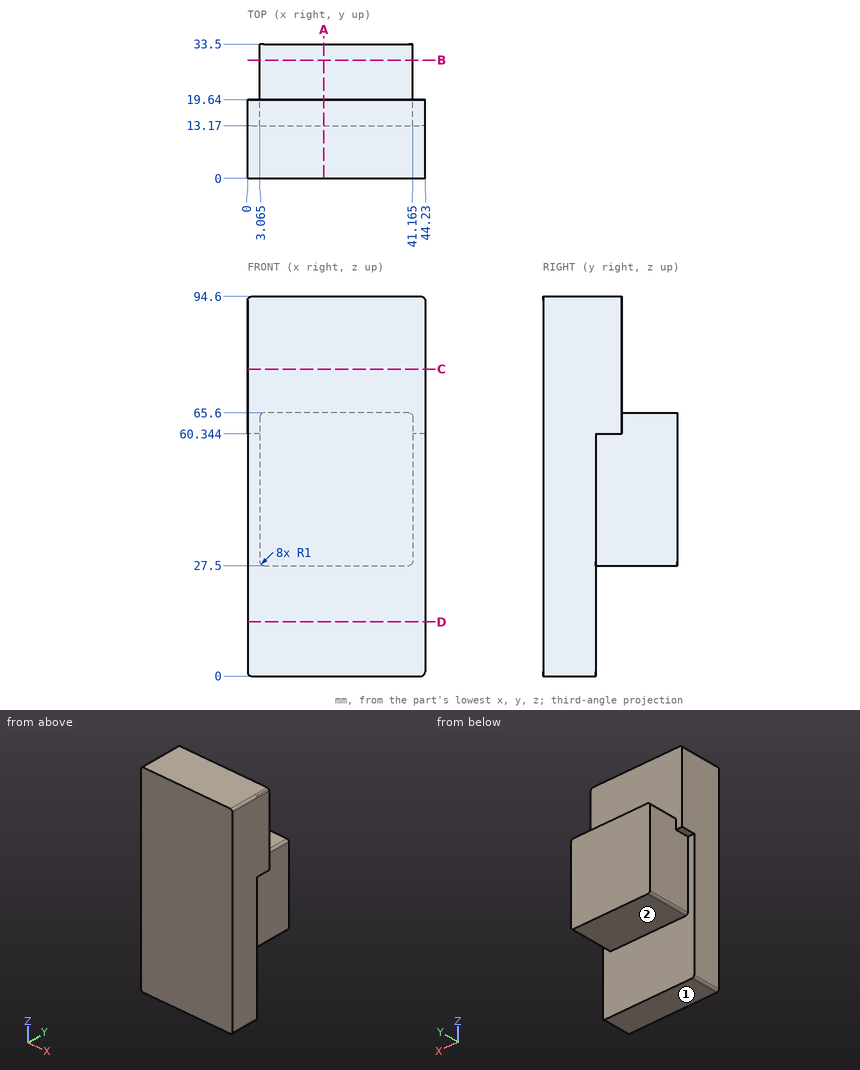
Geometry check sheet. Reference: drawing and pictorial views, mm from the part's lowest x, y, z. A direction names the side the tool comes from. Coordinates: 2 decimals unless noted, no trailing zeros. Order: outer loops, then holes, each group sorted by start corner. A loop starts at its lowest first (then second) coordinate and runs counter-clockwise, first axis right, second up.
Item 1: Material ranges on L1, parallel to Y at x = 35.5, z = 74; L2, parallel to X at y = 30.5, z = 47 (1 decimal); L3, parallel to Y at x = 24, z = 13.5, recorded low to high.
Filled in:
L1: y = 0 to 19.64
L2: x = 3.1 to 41.2
L3: y = 0 to 13.17
Item 2: Section check D-D, the plane z = 13.5. Enter the section's corners in (x, y).
Filled in:
outline: (0, 0) - (44.23, 0) - (44.23, 13.17) - (0, 13.17) - close
Item 3: Access from +Z, -Z, +X, -X, +Y, -Y to the whole of each face (thin tool, end or side, straight path). Record for the marked faces 1 and 2.
Filled in:
face 1: -Z, +X, -X, +Y, -Y
face 2: -Z, +X, -X, +Y
Item 4: Section check A-A, the plane x = 19. Enter the section's corners in (y, z), then the cut area to 3 significant figures.
Filled in:
outline: (0, 0) - (13.17, 0) - (13.17, 27.5) - (33.5, 27.5) - (33.5, 65.6) - (19.64, 65.6) - (19.64, 94.6) - (0, 94.6) - close
area: 2,210 mm2
Item 5: Section check B-B, the plane y = 29.5. Enter the section's corners in (x, z) (1 decimal).
Filled in:
outline: (3.1, 28.5) arc R1 ccw to (4.1, 27.5) - (40.2, 27.5) arc R1 ccw to (41.2, 28.5) - (41.2, 64.6) arc R1 ccw to (40.2, 65.6) - (4.1, 65.6) arc R1 ccw to (3.1, 64.6) - close
Item 6: Depth check by flat-ended pin: pin 1 (4 mm diameter, centred on y = 18.5, z = 83.5, fed in from -X); pin 2 (10 mm diameter, centred on y = 24.5, z = 47, fed in from +X) (1 decimal); pin 3 (3 mm diameter, centred on x = 25, y = 22.5, fed in from -Z); pin 4 (10 mm diameter, centred on y = 20.5, z = 40, fed in from -X) (1 decimal). Enter the tip coordinate at first touch or a pass-through.
Filled in:
pin 1: stops at x = 0
pin 2: stops at x = 41.2
pin 3: stops at z = 27.5
pin 4: stops at x = 3.1
Item 7: Section check C-C, the plane z = 76.5. Enter the section's corners in (x, y), then the cut area to 3 significant figures.
Filled in:
outline: (0, 0) - (44.23, 0) - (44.23, 19.64) - (0, 19.64) - close
area: 869 mm2
